```python
from build123d import *

# Parameters (mm, degrees)
EXTRUDE_1_DEPTH     = 297.016771
SKETCH_2_R          = 12.6
CUT_EXTRUDE_1_DEPTH = 31


with BuildPart() as part:
    # Эскиз1 → Бобышка-Вытянуть1 (new body)
    with BuildSketch(Plane(origin=(0, 0, 0), x_dir=(0, 0, -1), z_dir=(1, 0, 0))):
        with BuildLine():
            Line((-12, 15), (12, 15))
            ThreePointArc((12, 15), (14.121320344, 14.121320344), (15, 12))
            Line((15, 12), (15, -12))
            ThreePointArc((15, -12), (14.121320344, -14.121320344), (12, -15))
            Line((12, -15), (-12, -15))
            ThreePointArc((-12, -15), (-14.121320344, -14.121320344), (-15, -12))
            Line((-15, -12), (-15, 12))
            ThreePointArc((-15, 12), (-14.121320344, 14.121320344), (-12, 15))
        make_face()
        with BuildLine():
            Line((-11, 13), (11, 13))
            ThreePointArc((11, 13), (12.414213562, 12.414213562), (13, 11))
            Line((13, 11), (13, -11))
            ThreePointArc((13, -11), (12.414213562, -12.414213562), (11, -13))
            Line((11, -13), (-11, -13))
            ThreePointArc((-11, -13), (-12.414213562, -12.414213562), (-13, -11))
            Line((-13, -11), (-13, 11))
            ThreePointArc((-13, 11), (-12.414213562, 12.414213562), (-11, 13))
        make_face(mode=Mode.SUBTRACT)
    extrude(amount=-EXTRUDE_1_DEPTH)

    # Эскиз2 → Вырез-Вытянуть1 (cut, through all)
    with BuildSketch(Plane.XY.offset(15)):
        Circle(SKETCH_2_R)
    extrude(amount=-CUT_EXTRUDE_1_DEPTH, mode=Mode.SUBTRACT)


solid = part.part
```
Here's how the part is built. I have some questions about the finished solid (model axes, mm). A direction names the side the tool comes from. Round coordinates to 2 decimals unless told otherwise and drop trailing zeros. Loops run counter-clockwise (first coordinate to the right, second up) from the corner with the lowest first, then second, coordinate; pieces in that order, holes last.
1. If I drill on probe 1 along Z at (x, y) = (-177, 11); probe 2 along Z at (x, y) = (-56.5, -12.5), over which ranges is the centre line in solid material (lowest first)?
Answers:
probe 1: z = -15 to -13, 13 to 15
probe 2: z = -14.96 to -12.32, 12.32 to 14.96
2. Thinking about a two-plate mould opening in Y: for faces 1 (the face through (-12.597, 0.277, 13.931)), 2 (the face through (-148, 0, -15)), 3 (the face through (-146, -15, 0)), which applies, released by +Y, released by -Y, zero draft, split by the parting line, or undercut?
Answers:
face 1: undercut
face 2: zero draft
face 3: released by -Y
3. For faces 4 (the face through (-148, 0, 15)), 5 (the face through (-146, 13, 0)), which set-ups out of +Z, -Z, +X, -X, +Y, -Y let a thin tool reach every point of the face, with its end or its side?
Answers:
face 4: +Z, +X, -X, +Y, -Y
face 5: +X, -X
4. Suppose I cut it at A-A, the plane y = 0. Please give me the cut outline in (x, z), and give its area (3 significant figures).
Answers:
outline: (-297.02, -15) - (-12.6, -15) - (-12.6, -13) - (-297.02, -13) - close; (-297.02, 13) - (-12.6, 13) - (-12.6, 15) - (-297.02, 15) - close
area: 1,140 mm2
5. Suppose I cut it at B-B, the plane z = -7. Please give me the cut outline in (x, y), and give its area (3 significant figures).
Answers:
outline: (-297.02, -15) - (0, -15) - (0, -13) - (-297.02, -13) - close; (-297.02, 13) - (0, 13) - (0, 15) - (-297.02, 15) - close
area: 1,190 mm2
6. Suppose I cut it at C-C, the plane x = -189. Please give me the cut outline in (y, z).
Answers:
outline: (-15, -12) arc R3 ccw to (-12, -15) - (12, -15) arc R3 ccw to (15, -12) - (15, 12) arc R3 ccw to (12, 15) - (-12, 15) arc R3 ccw to (-15, 12) - close; hole (-13, -11) arc R2 ccw to (-11, -13) - (11, -13) arc R2 ccw to (13, -11) - (13, 11) arc R2 ccw to (11, 13) - (-11, 13) arc R2 ccw to (-13, 11) - close
